```python
from build123d import *

# Parameters (mm, degrees)
EXTRUDE_1_DEPTH          = 15
EXTRUDE_1_2_DEPTH        = 15
EXTRUDE_START            = 44.8
EXTRUDE_2_DEPTH          = 29.8
EXTRUDE_START_2          = -15
EXTRUDE_3_DEPTH          = 29.8
CUT_EXTRUDE_START        = 41.8
CUT_EXTRUDE_1_DEPTH      = 23.8
CUT_EXTRUDE_START_2      = -18
CUT_EXTRUDE_2_DEPTH      = 23.8
CUT_EXTRUDE_3_DEPTH      = 46.774337789
CUT_EXTRUDE_3_DEPTH_BACK = 46.774337789
SKETCH_4_R               = 1.1


with BuildPart() as part:
    # Sketch 1 → Extrude 1 (new, symmetric)
    with BuildSketch(Plane(origin=(0, 0, 0), x_dir=(0, 0, -1), z_dir=(1, 0, 0))):
        with BuildLine():
            Line((-3.291900756, 1.5), (3.291900756, 1.5))
            ThreePointArc((3.291900756, 1.5), (5.438638051, 3.682682292), (8.5, 3.708099244))
            Line((8.5, 3.708099244), (8.5, 2.598076211))
            ThreePointArc((8.5, 2.598076211), (5.722521613, 2.714415033), (4.041960108, 0.5))
            Line((4.041960108, 0.5), (-4.041960108, 0.5))
            ThreePointArc((-4.041960108, 0.5), (-5.722521613, 2.714415033), (-8.5, 2.598076211))
            Line((-8.5, 2.598076211), (-8.5, 3.708099244))
            ThreePointArc((-8.5, 3.708099244), (-5.438638051, 3.682682292), (-3.291900756, 1.5))
        make_face()
    extrude(amount=EXTRUDE_1_DEPTH, both=True)



with BuildPart() as body_2:
    # Sketch 1 → Extrude 1 2 (new, symmetric)
    with BuildSketch(Plane(origin=(0, 0, 0), x_dir=(0, 0, -1), z_dir=(1, 0, 0))):
        with BuildLine():
            Line((-3.291900756, -1.5), (3.291900756, -1.5))
            ThreePointArc((3.291900756, -1.5), (5.438638051, -3.682682292), (8.5, -3.708099244))
            Line((8.5, -3.708099244), (8.5, -2.598076211))
            ThreePointArc((8.5, -2.598076211), (5.722521613, -2.714415033), (4.041960108, -0.5))
            Line((4.041960108, -0.5), (-4.041960108, -0.5))
            ThreePointArc((-4.041960108, -0.5), (-5.722521613, -2.714415033), (-8.5, -2.598076211))
            Line((-8.5, -2.598076211), (-8.5, -3.708099244))
            ThreePointArc((-8.5, -3.708099244), (-5.438638051, -3.682682292), (-3.291900756, -1.5))
        make_face()
    extrude(amount=EXTRUDE_1_2_DEPTH, both=True)


with BuildPart() as part_1:
    add(part.part)

    add(body_2.part)  # Extrude 2 merges body 2
    # Sketch 2 → Extrude 2 (add)
    with BuildSketch(Plane(origin=(0, 0, 0), x_dir=(0, 0, -1), z_dir=(1, 0, 0)).offset(EXTRUDE_START)):
        with BuildLine():
            Line((-3.291900756, -1.5), (3.291900756, -1.5))
            ThreePointArc((3.291900756, -1.5), (5.438638051, -3.682682292), (8.5, -3.708099244))
            Line((8.5, -3.708099244), (8.5, 3.708099244))
            ThreePointArc((8.5, 3.708099244), (5.438638051, 3.682682292), (3.291900756, 1.5))
            Line((3.291900756, 1.5), (-3.291900756, 1.5))
            ThreePointArc((-3.291900756, 1.5), (-5.438638051, 3.682682292), (-8.5, 3.708099244))
            Line((-8.5, 3.708099244), (-8.5, -3.708099244))
            ThreePointArc((-8.5, -3.708099244), (-5.438638051, -3.682682292), (-3.291900756, -1.5))
        make_face()
    extrude(amount=-EXTRUDE_2_DEPTH)

    # Sketch 2_2 → Extrude 3 (add)
    with BuildSketch(Plane(origin=(0, 0, 0), x_dir=(0, 0, -1), z_dir=(1, 0, 0)).offset(EXTRUDE_START_2)):
        with BuildLine():
            Line((-3.291900756, -1.5), (3.291900756, -1.5))
            ThreePointArc((3.291900756, -1.5), (5.438638051, -3.682682292), (8.5, -3.708099244))
            Line((8.5, -3.708099244), (8.5, 3.708099244))
            ThreePointArc((8.5, 3.708099244), (5.438638051, 3.682682292), (3.291900756, 1.5))
            Line((3.291900756, 1.5), (-3.291900756, 1.5))
            ThreePointArc((-3.291900756, 1.5), (-5.438638051, 3.682682292), (-8.5, 3.708099244))
            Line((-8.5, 3.708099244), (-8.5, -3.708099244))
            ThreePointArc((-8.5, -3.708099244), (-5.438638051, -3.682682292), (-3.291900756, -1.5))
        make_face()
    extrude(amount=-EXTRUDE_3_DEPTH)

    # Sketch 3 → Cut-Extrude 1 (cut)
    with BuildSketch(Plane(origin=(0, 0, 0), x_dir=(0, 0, -1), z_dir=(1, 0, 0)).offset(CUT_EXTRUDE_START)):
        with BuildLine():
            Line((-4.041960108, 0.5), (-4.041960108, -0.5))
            ThreePointArc((-4.041960108, -0.5), (-5.722521613, -2.714415033), (-8.5, -2.598076211))
            Line((-8.5, -2.598076211), (-8.5, 2.598076211))
            ThreePointArc((-8.5, 2.598076211), (-5.722521613, 2.714415033), (-4.041960108, 0.5))
        make_face()
        with BuildLine():
            Line((8.5, 2.598076211), (8.5, -2.598076211))
            ThreePointArc((8.5, -2.598076211), (5.722521613, -2.714415033), (4.041960108, -0.5))
            Line((4.041960108, -0.5), (4.041960108, 0.5))
            ThreePointArc((4.041960108, 0.5), (5.722521613, 2.714415033), (8.5, 2.598076211))
        make_face()
    extrude(amount=-CUT_EXTRUDE_1_DEPTH, mode=Mode.SUBTRACT)

    # Sketch 3_2 → Cut-Extrude 2 (cut)
    with BuildSketch(Plane(origin=(0, 0, 0), x_dir=(0, 0, -1), z_dir=(1, 0, 0)).offset(CUT_EXTRUDE_START_2)):
        with BuildLine():
            Line((-4.041960108, 0.5), (-4.041960108, -0.5))
            ThreePointArc((-4.041960108, -0.5), (-5.722521613, -2.714415033), (-8.5, -2.598076211))
            Line((-8.5, -2.598076211), (-8.5, 2.598076211))
            ThreePointArc((-8.5, 2.598076211), (-5.722521613, 2.714415033), (-4.041960108, 0.5))
        make_face()
        with BuildLine():
            Line((8.5, 2.598076211), (8.5, -2.598076211))
            ThreePointArc((8.5, -2.598076211), (5.722521613, -2.714415033), (4.041960108, -0.5))
            Line((4.041960108, -0.5), (4.041960108, 0.5))
            ThreePointArc((4.041960108, 0.5), (5.722521613, 2.714415033), (8.5, 2.598076211))
        make_face()
    extrude(amount=-CUT_EXTRUDE_2_DEPTH, mode=Mode.SUBTRACT)

    # Sketch 4 → Cut-Extrude 3 (cut, two sides: drawn at the far end of the back side and taken through both)
    with BuildSketch(Plane(origin=(0, 0, 0), x_dir=(0, 0, -1), z_dir=(1, 0, 0)).offset(-CUT_EXTRUDE_3_DEPTH_BACK)):
        with Locations((-7, 0)):
            Circle(SKETCH_4_R)
        with Locations((7, 0)):
            Circle(SKETCH_4_R)
    extrude(amount=CUT_EXTRUDE_3_DEPTH + CUT_EXTRUDE_3_DEPTH_BACK, mode=Mode.SUBTRACT)


solid = part_1.part
```
CAD build for the part. Positions are in the model's coordinates, mm. A direction names the side the tool comes from. Round coordinates to 2 decimals unless told otherwise and drop trailing zeros. Order: outer loops, then holes, each group sorted by start corner. A loop starts at its lowest first (then second) coordinate and runs counter-clockwise, first axis right, second up. Notation, with made-up numbers: (54, 44) -> (109, 44) arc R19 cw to (109, 63) -> close; hole circle Ø10 at (42.5, -32). An arc over 180 degrees is marked (long way). Write item = value, one per line.
(1) Pull direction Z, two halves, no side cores. Call faces 1 (the flat face through (44.8, 0, 0)), 2 (the flat face through (0, -3, -8.5)), 3 (the cylindrical face through (43.279, -0.421, 5.984)): +Z half, -Z half, draft (parallel to the pull), parting line (faces both ways), or undercut.
Answers follow:
face_1 = draft
face_2 = -Z half
face_3 = undercut
(2) Cut at B-B (z = -1). Write the cut outline in (x, y), plus the area to 3 significant figures.
Answers follow:
outline = (-44.8, -1.5) -> (44.8, -1.5) -> (44.8, 1.5) -> (-44.8, 1.5) -> close; hole (-15, -0.5) -> (15, -0.5) -> (15, 0.5) -> (-15, 0.5) -> close
area = 239 mm²
(3) Flat gauge pins, fed straight in: P1, Ø3.5, axis at x = 10.5, z = 1.5, coming from the +Y side; P2, Ø7, axis at x = -18.5, z = -0.5, coming from the -Y side; P3, Ø6, axis at x = -22.5, z = 2, coming from the +Y side. Where does each tip first touch, or does it go through?
Answers follow:
P1 = 1.5
P2 = -2.65
P3 = 3.46
(4) Cut at C-C (x = 23). Write the cut outline in (y, z).
Answers follow:
outline = (-3.71, -8.5) -> (-2.6, -8.5) arc R3 cw to (-0.5, -4.04) -> (0.5, -4.04) arc R3 cw to (2.6, -8.5) -> (3.71, -8.5) arc R4 ccw to (1.5, -3.29) -> (1.5, 3.29) arc R4 ccw to (3.71, 8.5) -> (2.6, 8.5) arc R3 cw to (0.5, 4.04) -> (-0.5, 4.04) arc R3 cw to (-2.6, 8.5) -> (-3.71, 8.5) arc R4 ccw to (-1.5, 3.29) -> (-1.5, -3.29) arc R4 ccw to start
(5) 3-axis set-ups, long thin cutter, end or side, ignore diameter. For faces 4 (the flat face through (0, 0.5, 0)), 5 (the cylindrical face through (0.21, -2.73, -5.76)), 6 (the flat face through (1, 1.5, 0)): which of +Z, -Z, +X, -X, +Y, -Y reach the whole face in a straight line?
Answers follow:
face_4 = +Z, -Z
face_5 = none
face_6 = +X, -X, +Y
(6) Drill centre lines: L1, parallel to Z at x = 16.35, y = 0; L2, parallel to X at y = -1.25, z = -6; L3, parallel to Y at x = -6, z = 0. Where is each one in solid material? Low to high.
Answers follow:
L1 = -8.5 to -8.1, -5.9 to 5.9, 8.1 to 8.5
L2 = -44.8 to -41.8, -18 to -15, 15 to 18, 41.8 to 44.8
L3 = -1.5 to -0.5, 0.5 to 1.5
